Autodesk Inventor part; units mm, degrees
ref_plane "YZ Plane" through (0, 0, 0) normal (1, 0, 0) x (0, 1, 0)
ref_plane "XZ Plane" through (0, 0, 0) normal (0, 1, 0) x (-1, 0, 0)
ref_plane "XY Plane" through (0, 0, 0) normal (0, 0, 1) x (1, 0, 0)
sketch "Sketch2" plane through (0, 0, 0) normal (0, 0, 1) x (1, 0, 0)
  line L0 (0, 76.4315) -> (0, -76.4315) construction
  arc A0 (-39.5643, 82.3191) -> (39.5643, 82.3191) centre (0, 76.4315) ccw construction
  arc A1 (61.8193, -67.2321) -> (-61.8193, -67.2321) centre (0, -76.4315) ccw construction
  line L1 (61.8193, -67.2321) -> (39.5643, 82.3191)
  line L2 (-61.8193, -67.2321) -> (-39.5643, 82.3191)
  arc A2 (39.5643, 82.3191) -> (-39.5643, 82.3191) centre (0, 76.4315) ccw
  arc A3 (-61.8193, -67.2321) -> (61.8193, -67.2321) centre (0, -76.4315) ccw
  line L3 (0, 76.4315) -> (0, 116.4315) construction
  point P0 (0, 0)
  point P1 (0, 0)
  dimension "d1" = 152.863
  dimension "d2" = 80
  dimension "d3" = 125
sketch "Sketch3" plane through (0, 0, 0) normal (1, 0, 0) x (0, 1, 0)
  line L0 (118.9301, 0) -> (112.9301, 0) construction
  line L1 (116.4315, 4.25) -> (116.4315, -4.25) construction
  line L2 (118.9301, 5.1594) -> (118.9301, -5.1594)
  line L3 (118.9301, -5.1594) -> (112.9301, -2.9756)
  line L4 (112.9301, -2.9756) -> (112.9301, 2.9756)
  line L5 (112.9301, 2.9756) -> (118.9301, 5.1594)
  point P0 (0, 0)
  point P1 (0, 0)
  point P2 (116.4315, 0)
  point P3 (116.4315, 0)
  point P4 (116.4315, 0)
  dimension "d4" = 8.5
  dimension "d5" = 2.4986
  dimension "d6" = 40
  dimension "d7" = 6
sweep "Sweep1" add profiles "Sketch3" path "Sketch2"
equation "\"d4\" = d8"
equation "\"d5\" = d9"
equation "\"d6\" = d10"
equation "\"d7\" = d11"
equation "\"d8\" = 8.5"
equation "\"d9\" = 2.49859"
equation "\"d10\" = 40deg"
equation "\"d11\" = 6"
properties part number "PWTR-0097" material "Rubber"
The model under review builds one solid part; all positions refer to its coordinate system, in mm. A direction names the side the tool comes from. Coordinates: 2 decimals unless noted, no trailing zeros. Write each loop counter-clockwise with the first axis right and the second up, starting at its lowest first coordinate (ties: lowest second). Pieces come first, ordered by that corner, then holes. Notation, with made-up numbers: (-27, 24) -> (-9, 24) arc R20 ccw to (-9, 42) -> close; hole circle Ø10 at (-4, 12.5). An arc over 180 degrees is marked (long way). Answer in a Markdown table with one row per item.
1. Clearance check with flat-ended pins moving along their axes: pin 1 Ø3 at (x, z) = (-45, -0.5) entering from -Y; pin 2 Ø3 at (x, z) = (10.5, -1) entering from +Y; pin 3 Ø5 at (x, z) = (1.5, -2) entering from +Y. State where each tip first meets the part, or that it passes through.
Answers below:
| item | result |
|---|---|
| pin 1 | stops at y = -124.73 |
| pin 2 | stops at y = 117.97 |
| pin 3 | stops at y = 118.93 |
2. Draft analysis for pull direction X (two halves, no side actions). For faces 5 (the flat face through (47.073, 8.075, 0.042)), 6 (the flat face through (50.08, 8.52, 4.08)), 7 (the flat face through (-53.32, 6.86, -0.07)), 8 (the cylindrical face through (0.85, 118.92, 0.07)), state which applies: +X half, -X half, draft (parallel to the pull), parting line (faces both ways), or undercut.
Answers below:
| item | result |
|---|---|
| face 5 | undercut |
| face 6 | undercut |
| face 7 | -X half |
| face 8 | parting line |
3. We need section C-C, the plane y = -7. State the section outline as (x, z) points.
Answers below:
| item | result |
|---|---|
| outline | (-55.38, -5.16) -> (-49.32, -2.98) -> (-49.32, 2.98) -> (-55.38, 5.16) -> close; (49.32, -2.98) -> (55.38, -5.16) -> (55.38, 5.16) -> (49.32, 2.98) -> close |
4. Wall thickness on probe 1 along Y at (x, z) = (-1, -2.75); probe 2 along X at (y, z) = (49.5, 2); probe 3 along X at (y, z) = (44.5, 2): over which ranges is each line inside the solid? List them lowest first. Write a range as [from, to].
Answers below:
| item | result |
|---|---|
| probe 1 | y = [-141.42, -135.42], [112.92, 118.92] |
| probe 2 | x = [-46.97, -40.91], [40.91, 46.97] |
| probe 3 | x = [-47.72, -41.65], [41.65, 47.72] |
5. We need section A-A, the plane x = 0. State the section outline as (y, z) points.
Answers below:
| item | result |
|---|---|
| outline | (-141.43, -5.16) -> (-135.43, -2.98) -> (-135.43, 2.98) -> (-141.43, 5.16) -> close; (112.93, -2.98) -> (118.93, -5.16) -> (118.93, 5.16) -> (112.93, 2.98) -> close |
6. For faces 1 (the flat face through (53, 9, 0)), 2 (the conical face through (1.428, -135.788, -3.112)), 3 (the cylindrical face through (-0.727, 112.923, -0.042)), 4 (the conical face through (0.735, 113.298, 3.112)), list the 3-axis set-ups (+Z, -Z, +X, -X, +Y, -Y) from which the entire face can be reached by the end or side of a thin tool; tool diameter is ignored.
Answers below:
| item | result |
|---|---|
| face 1 | +Z, -Z, +X, +Y |
| face 2 | -Z |
| face 3 | +Z, -Z |
| face 4 | +Z |
7. We need section B-B, the plane z = -0.25. State the section outline as (x, y) points, and give its area (3 significant figures).
Answers below:
| item | result |
|---|---|
| outline | (-64.29, -66.86) arc R65 ccw (long way) to (64.29, -66.86) -> (42.04, 82.69) arc R42.5 ccw to (-42.04, 82.69) -> close; hole (-58.36, -67.75) arc R59 ccw (long way) to (58.36, -67.75) -> (36.1, 81.8) arc R36.5 ccw to (-36.1, 81.8) -> close |
| area | 3,770 mm^2 |
